Can you work these out from the model? Positions are in its coordinate system, mm. A direction names the side the tool comes from. Coordinates: 2 decimals unless noted, no trailing zeros. Loops run counter-clockwise (first coordinate to the right, second up) from the corner with the lowest first, then second, coordinate; pieces in that order, holes last.
```python
from build123d import *

# Parameters (mm, degrees)
BOSS_EXTRUDE1_DEPTH         = 30
SKETCH2_W                   = 1
SKETCH2_H                   = 5
CUT_EXTRUDE1_DEPTH          = 300
SKETCH11_W                  = 100
SKETCH11_H                  = 14
SKETCH11_H_2                = 12.5
BOSS_EXTRUDE2_DEPTH         = 10
SKETCH3_R                   = 3
CUT_EXTRUDE2_DEPTH          = 100
SKETCH4_R                   = 7
CUT_EXTRUDE3_DEPTH          = 70
LPATTERN1_COUNT             = 2
LPATTERN1_PITCH             = 40
SKETCH9_R                   = 3.381759822
CUT_EXTRUDE8_DEPTH          = 100
CUT_EXTRUDE9_START          = -10
SKETCH10_R                  = 6.982534733
CUT_EXTRUDE9_DEPTH          = 20
LPATTERN4_COUNT             = 2
LPATTERN4_PITCH             = 140
SKETCH7_R                   = 2.900161541
CUT_EXTRUDE6_DEPTH          = 40
SKETCH8_R                   = 5.870976625
CUT_EXTRUDE7_DEPTH          = 25
PATTERN_LINEAR_1_COUNT      = 2
PATTERN_LINEAR_1_PITCH      = 40
PATTERN_LINEAR_1_COUNT_DIR2 = 2
PATTERN_LINEAR_1_PITCH_DIR2 = 113
SKETCH_1_W                  = 1
SKETCH_1_H                  = 5
CUT_EXTRUDE_1_DEPTH         = 200
CHAMFER_1_SIZE              = 1
SKETCH_3_R                  = 40
CUT_EXTRUDE_3_DEPTH         = 30
FILLET_1_R                  = 3


with BuildPart() as part:
    # Sketch1 → Boss-Extrude1 (new body)
    with BuildSketch(Plane.XY):
        Polygon((-23.103448276, -43.572275418), (-23.103448276, -8.572275418), (46.896551724, -8.572275418), (46.896551724, 52.427724582), (-23.103448276, 52.427724582), (-23.103448276, 136.427724582), (76.896551724, 136.427724582), (76.896551724, -43.572275418), align=None)
    extrude(amount=BOSS_EXTRUDE1_DEPTH)

    # Sketch2 → Cut-Extrude1 (cut)
    with BuildSketch(Plane.ZY.offset(23.103448276)):
        Polygon((30, 5.791685612), (23.636038969, -0.572275418), (23.636038969, -0.672275418), (30, -7.036236449), align=None)
        Polygon((30, 70.791685612), (23.636038969, 64.427724582), (22.636038969, 64.427724582), (22.636038969, 60.427724582), (23.636038969, 60.427724582), (30, 54.063763551), align=None)
        with Locations((29.5, -27.072275418)):
            Rectangle(SKETCH2_W, SKETCH2_H)
    extrude(amount=-CUT_EXTRUDE1_DEPTH, mode=Mode.SUBTRACT)

    # Sketch11 → Boss-Extrude2 (add)
    with BuildSketch(Plane.XY.offset(30)):
        with Locations((26.896551724, -36.572275418)):
            Rectangle(SKETCH11_W, SKETCH11_H)
        with Locations((26.896551724, 76.677724582)):
            Rectangle(SKETCH11_W, SKETCH11_H_2)
    extrude(amount=BOSS_EXTRUDE2_DEPTH)

    # Sketch3 → Cut-Extrude2 (cut)
    with BuildSketch(Plane(origin=(0, 136.427724582, 0), x_dir=(1, 0, 0), z_dir=(0, 1, 0))):
        with Locations(Location((-12.103448276, -15, 0), (0, 0, 270))):
            Circle(SKETCH3_R)
    cut_extrude2 = extrude(amount=-CUT_EXTRUDE2_DEPTH, mode=Mode.SUBTRACT)

    # Sketch4 → Cut-Extrude3 (cut)
    with BuildSketch(Plane(origin=(0, 136.427724582, 0), x_dir=(1, 0, 0), z_dir=(0, 1, 0))):
        with Locations(Location((-12.103448276, -15, 0), (0, 0, 270))):
            Circle(SKETCH4_R)
    cut_extrude3 = extrude(amount=-CUT_EXTRUDE3_DEPTH, mode=Mode.SUBTRACT)

    # LPattern1: Cut-Extrude2, Cut-Extrude3 ×2
    with Locations(*[(i * LPATTERN1_PITCH, 0, 0) for i in range(1, LPATTERN1_COUNT)]):
        add(cut_extrude2, mode=Mode.SUBTRACT)
        add(cut_extrude3, mode=Mode.SUBTRACT)

    # Sketch9 → Cut-Extrude8 (cut)
    with BuildSketch(Plane(origin=(0, 0, 0), x_dir=(-1, 0, 0), z_dir=(0, 0, -1))):
        with Locations((-66.896551724, 116.427724582)):
            Circle(SKETCH9_R)
    cut_extrude8 = extrude(amount=-CUT_EXTRUDE8_DEPTH, mode=Mode.SUBTRACT)

    # Sketch10 → Cut-Extrude9 (cut)
    with BuildSketch(Plane.XY.offset(30).offset(CUT_EXTRUDE9_START)):
        with Locations((66.896551724, 116.427724582)):
            Circle(SKETCH10_R)
    cut_extrude9 = extrude(amount=-CUT_EXTRUDE9_DEPTH, mode=Mode.SUBTRACT)

    # LPattern4: Cut-Extrude8, Cut-Extrude9 ×2
    with Locations(*[(-i * LPATTERN4_PITCH, 0, 0) for i in range(1, LPATTERN4_COUNT)]):
        add(cut_extrude8, mode=Mode.SUBTRACT)
        add(cut_extrude9, mode=Mode.SUBTRACT)

    # Sketch7 → Cut-Extrude6 (cut)
    with BuildSketch(Plane(origin=(0, 0, 0), x_dir=(-1, 0, 0), z_dir=(0, 0, -1))):
        with Locations((-1.896551724, -36.572275418)):
            Circle(SKETCH7_R)
    cut_extrude6 = extrude(amount=-CUT_EXTRUDE6_DEPTH, mode=Mode.SUBTRACT)

    # Sketch8 → Cut-Extrude7 (cut)
    with BuildSketch(Plane(origin=(0, 0, 0), x_dir=(-1, 0, 0), z_dir=(0, 0, -1))):
        with Locations((-1.896551724, -36.572275418)):
            Circle(SKETCH8_R)
    cut_extrude7 = extrude(amount=-CUT_EXTRUDE7_DEPTH, mode=Mode.SUBTRACT)

    # Линейный массив1: Cut-Extrude6, Cut-Extrude7 2 × 2
    with Locations(*[(i * PATTERN_LINEAR_1_PITCH, j * PATTERN_LINEAR_1_PITCH_DIR2, 0) for i in range(PATTERN_LINEAR_1_COUNT) for j in range(PATTERN_LINEAR_1_COUNT_DIR2) if (i, j) != (0, 0)]):
        add(cut_extrude6, mode=Mode.SUBTRACT)
        add(cut_extrude7, mode=Mode.SUBTRACT)

    # Эскиз1 → Вырез-Вытянуть1 (cut)
    with BuildSketch(Plane.ZY.offset(23.103448276)):
        with Locations((29.5, 85.427724582)):
            Rectangle(SKETCH_1_W, SKETCH_1_H)
    extrude(amount=-CUT_EXTRUDE_1_DEPTH, mode=Mode.SUBTRACT)

    # Фаска1
    chamfer_1_edges = [part.edges().sort_by_distance(p)[0] for p in [
        (26.896551724, 70.427724582, 40),
        (26.896551724, -29.572275418, 40),
    ]]
    chamfer(chamfer_1_edges, length=CHAMFER_1_SIZE)

    # Эскиз3 → Вырез-Вытянуть3 (cut)
    with BuildSketch(Plane.XZ.offset(43.572275418)):
        with Locations((-59.800747668, -15)):
            Circle(SKETCH_3_R)
    extrude(amount=-CUT_EXTRUDE_3_DEPTH, mode=Mode.SUBTRACT)

    # Скругление1
    # the kernel refuses this fillet: 3 mm, written as the material it takes off along each edge
    with BuildSketch(Plane(origin=(-22.719755232, -13.572275418, 0), x_dir=(-0.3864755051047792, 0, 0.9222996714484971), z_dir=(0, -1, 0))) as fillet_1_piece_1:
        with BuildLine():
            CenterArc((2.081301731, -2.795561642), FILLET_1_R, 111.274329899, 45.990298087)
            Line((-0.685597284, -1.636135127), (-0.740935264, -1.612946597))
            Line((-0.740935264, -1.612946597), (-0.05533798, 0.02318853))
            Line((-0.05533798, 0.02318853), (0.0007446, 0.05999538))
            ThreePointArc((0.0007446, 0.05999538), (0.49640021, 0.056919717), (0.971030393, 0.055911233))
            Line((0.971030393, 0.055911233), (0.992800419, 0))
        make_face()
    extrude(amount=34.434933616, mode=Mode.SUBTRACT)


solid = part.part
```
Item 1: On a 3-axis mill with a long thin cutter (end or side, diameter ignored), from which of +Z, -Z, +X, -X, +Y, -Y can I reach the whole of each face in a straight line? I mean faces 4 (the face through (12, 52.428, 15)), 5 (the face through (-16.363, 101.918, 9.445)), 6 (the face through (3.169, -42.304, 12.325)), 7 (the face through (26.197, 57.29, 26.773)). Say none if no direction works.
Results are:
face 4: +Z, -Z, -X
face 5: +Y
face 6: -Z
face 7: +Z, +X, -X
Item 2: We'd pull the mould along Z, two halves only. Please class faces 1 (the face through (26, 62, 22.636)), 2 (the face through (46.897, 22, 15)), 3 (the face through (-15.1, 66.428, 16.5)): +Z half, -Z half, draft (parallel to the pull), parting line (faces both ways), or undercut.
Results are:
face 1: +Z half
face 2: draft
face 3: undercut
Item 3: I need wall thicknesses on line 1 along X through (y, z) = (59.5, 15); line 2 along Y through (x, z) = (47, 6); line 3 along Y through (x, z) = (-17, 16). Which ranges of each line are inside material? Lowest first, please.
Results are:
line 1: x = -23.1 to -15.1, -9.1 to 24.9, 30.9 to 76.9
line 2: y = -43.57 to -39.47, -33.67 to 73.53, 79.33 to 136.43
line 3: y = -43.57 to -8.57, 52.43 to 66.43
Item 4: Suppose I cut it at B-B, the plane x = 51. Please give me the cut outline in (y, z), plus the area to 3 significant figures.
Results are:
outline: (-43.57, 0) - (136.43, 0) - (136.43, 30) - (87.93, 30) - (87.93, 29) - (82.93, 29) - (82.93, 40) - (71.43, 40) - (70.43, 39) - (70.43, 30) - (70.79, 30) - (64.43, 23.64) - (64.43, 22.64) - (60.43, 22.64) - (60.43, 23.64) - (54.06, 30) - (5.79, 30) - (-0.57, 23.64) - (-0.67, 23.64) - (-7.04, 30) - (-24.57, 30) - (-24.57, 29) - (-29.57, 29) - (-29.57, 39) - (-30.57, 40) - (-43.57, 40) - close
area: 5,540 mm2
Item 5: Suppose I cut it at A-A, the plane z = 16. Count the separate pieces of the cut face and the enclosed holes in it, plus the area to 3 significant figures.
Results are:
separate pieces: 3
enclosed holes: 5
area: 11,000 mm2
Item 6: Suppose I cut it at C-C, the plane z = 27. Please give me the cut outline in (x, y), plus the area to 3 significant figures.
Results are:
outline: (-23.1, -43.57) - (76.9, -43.57) - (76.9, -4.04) - (46.9, -4.04) - (46.9, -8.57) - (-23.1, -8.57) - close; (-23.1, 52.43) - (46.9, 52.43) - (46.9, 2.79) - (76.9, 2.79) - (76.9, 57.06) - (-23.1, 57.06) - close; (-23.1, 67.79) - (76.9, 67.79) - (76.9, 136.43) - (-23.1, 136.43) - close; hole circle Ø5.8 at (1.9, -36.57); hole circle Ø5.8 at (1.9, 76.43); hole circle Ø5.8 at (41.9, -36.57); hole circle Ø5.8 at (41.9, 76.43); hole circle Ø6.76 at (66.9, 116.43)
area: 12,300 mm2
Item 7: I'm going to push flat-ended pins straight in: P1, Ø1.5, axis at x = 58, y = 8, coming from the +Z side; P2, Ø1.5, axis at x = 30.5, y = -28, coming from the +Z side; P3, Ø5, axis at x = 41.9, y = -36.57, coming from the -Z side; P4, Ø9, axis at y = 29.5, z = 21, coming from the -X side. Where does each tip first touch, or does it pass through?
Results are:
P1: stops at z = 30
P2: stops at z = 29
P3: passes through
P4: stops at x = 46.9
